Could you check a few things on this model? Use its own coordinates, in mm. Face numbers are marked on the shaded views. Round coordinates to 2 decimals unless told otherwise and drop trailing zeros. Write each loop counter-clockwise with the first axis right and the second up, starting at its lowest first coordinate (ties: lowest second). Pieces come first, ordered by that corner, then holes. Notation, with made-up numbers: (-2, 62.5) -> (32, 62.5) arc R15 cw to (32, 79.5) -> close; hole circle Ø4 at (61.25, 55). An arc over 180 degrees is marked (long way). Answer as CSV lines item,"result". Start each with the question number.
Q1. If I drill on line 1 (Y direction, x = -15.5, z = -14.5); line 2 (X direction, y = 8.75, z = -8); line 3 (Z direction, x = -18, y = 11.75), over which ranges is the centre line in solid material (lowest first)? Write a range as [from, to].
Q2. Will these pins go through, and if not, where does the flat tip stop? pin 1 Ø2 at (x, y) = (-8, 8.5) entering from -Z; pin 2 Ø1.9 at (y, z) = (-0.5, -1.5) entering from +X; pin 3 Ø18 at (x, z) = (0, 0) entering from +Y; pin 4 Ø2.5 at (x, z) = (8.84, 8.84) entering from -Y.
Q3. Imagine slicing it at A-A on z = 0. Please give me the cut outline in (x, y), and give its area (3 significant figures).
Q4. Imagine slicing it at C-C on y = 14.75. Please give me the cut outline in (x, z).
Q5. Imagine slicing it at B-B on x = 0. Please give me the cut outline in (y, z).
Q6. If we mould it in two halves opening along X, with no side actions, what happens to the marked faces 1, 2 and 3? For each: pulls with the +X half, pulls with the -X half, needs draft (parallel to the pull), parting line crosses it, or undercut.
from build123d import *
from build123d.topology import SkipClean

# Parameters (mm, degrees)
SKETCH_1_R          = 26
SKETCH_1_R_2        = 24
EXTRUDE_1_DEPTH     = 26
EXTRUDE_START       = 1
SKETCH_2_R          = 26
EXTRUDE_2_DEPTH     = 1
CUT_EXTRUDE_4_REACH = 47.033
FILLET_2_R          = 4
EXTRUDE_START_2     = 0.7
EXTRUDE_3_DEPTH     = 0.7
CUT_EXTRUDE_1_REACH = 48.036
SKETCH_4_R          = 7
HOLE_WIZARD_M31_D   = 3.4
CHAMFER_1_SIZE      = 0.5


with BuildPart() as part:
    # Эскиз1 → Бобышка-Вытянуть1 (new body)
    with BuildSketch(Plane(origin=(0, 0, 0), x_dir=(1, 0, 0), z_dir=(0, 1, 0))):
        with Locations(Location((0, 0, 0), (0, 0, 90))):
            Circle(SKETCH_1_R)
        with Locations(Location((0, 0, 0), (0, 0, 90))):
            Circle(SKETCH_1_R_2, mode=Mode.SUBTRACT)
    extrude(amount=EXTRUDE_1_DEPTH)

    # Эскиз2 → Бобышка-Вытянуть2 (add)
    with BuildSketch(Plane.XZ.offset(EXTRUDE_START)):
        with Locations(Location((0, 0, 0), (0, 0, 270))):
            Circle(SKETCH_2_R)
    extrude(amount=-EXTRUDE_2_DEPTH)

    # Эскиз9 → Вырез-Вытянуть4 (cut, up to next)
    with BuildSketch(Plane(origin=(0, 0, 0), x_dir=(1, 0, 0), z_dir=(0, 1, 0)), mode=Mode.PRIVATE) as cut_extrude_4_sk1:
        with BuildLine():
            Line((15, 18.734993995), (15, -18.734993995))
            ThreePointArc((15, -18.734993995), (24, 0), (15, 18.734993995))
        make_face()
    cut_extrude_4_tool1 = extrude(cut_extrude_4_sk1.sketch, amount=-CUT_EXTRUDE_4_REACH, mode=Mode.PRIVATE) & part.part
    add(cut_extrude_4_tool1.solids().sort_by_distance((18.66496, 0, 0))[0], mode=Mode.SUBTRACT)

    # Скругление2
    fillet_2_edges = [part.edges().sort_by_distance(p)[0] for p in [
        (15, -0.5, -18.734993995),
        (15, -0.5, 18.734993995),
    ]]
    fillet(fillet_2_edges, radius=FILLET_2_R)

    # Эскиз3 → Бобышка-Вытянуть3 (add)
    with SkipClean():  # the faces are left unmerged after this step: merging them gives an invalid solid
        with BuildSketch(Plane.XZ.offset(1).offset(EXTRUDE_START_2)):
            with BuildLine():
                Line((15, -6.244997998), (15, 6.244997998))
                ThreePointArc((15, 6.244997998), (16.303590006, 9.199549257), (19.364686571, 10.22833877))
                ThreePointArc((19.364686571, 10.22833877), (-21.9, 0), (19.364686571, -10.22833877))
                ThreePointArc((19.364686571, -10.22833877), (16.303590006, -9.199549257), (15, -6.244997998))
            make_face()
        extrude(amount=-EXTRUDE_3_DEPTH)

    # Эскиз4 → Вырез-Вытянуть1 (cut, up to next)
    with BuildSketch(Plane.XZ.offset(1.7), mode=Mode.PRIVATE) as cut_extrude_1_sk1:
        with Locations(Location((0, 0, 0), (0, 0, 270))):
            Circle(SKETCH_4_R)
    cut_extrude_1_tool1 = extrude(cut_extrude_1_sk1.sketch, amount=-CUT_EXTRUDE_1_REACH, mode=Mode.PRIVATE) & part.part
    add(cut_extrude_1_tool1.solids().sort_by_distance((0, -1.7, 0))[0], mode=Mode.SUBTRACT)

    # Отверстие с зазором M31 (through all)
    with Locations(Plane(origin=(0, -1.7, 0), x_dir=(-1, 0, 0), z_dir=(0, -1, 0))):
        with Locations((8.838834765, -8.838834765), (-8.838834765, -8.838834765), (-8.838834765, 8.838834765), (8.838834765, 8.838834765)):
            Hole(HOLE_WIZARD_M31_D / 2)

    # Фаска1
    chamfer_1_edges = [part.edges().sort_by_distance(p)[0] for p in [
        (0, -1, 26),
    ]]
    chamfer(chamfer_1_edges, length=CHAMFER_1_SIZE)


solid = part.part
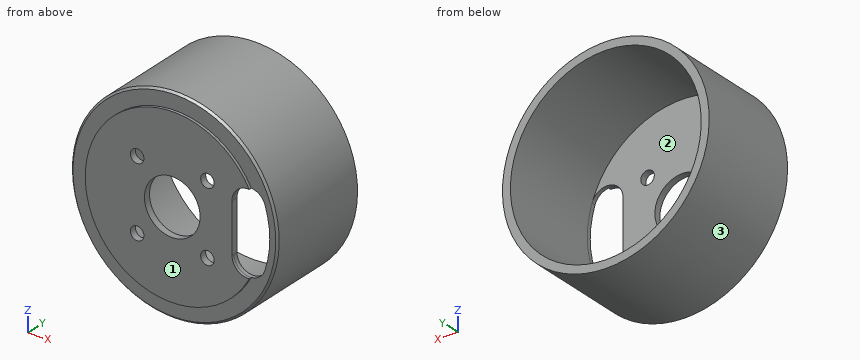
Checks:
1,line 1,"[-1.7, 0]"
1,line 2,"[-24.74, -22.63], [22.63, 24.74]"
1,line 3,"[-18.76, -15.87], [15.87, 18.76]"
2,pin 1,"z = -25.04"
2,pin 2,"x = 25.99"
2,pin 3,"y = 0"
2,pin 4,"through"
3,outline,"(-26, -0.5) -> (-25.5, -1) -> (-21.9, -1) -> (-21.9, -1.7) -> (-7, -1.7) -> (-7, 0) -> (-24, 0) -> (-24, 26) -> (-26, 26) -> close; (7, -1.7) -> (15, -1.7) -> (15, 0) -> (7, 0) -> close; (24, -1) -> (25.5, -1) -> (26, -0.5) -> (26, 26) -> (24, 26) -> close"
3,area,"149 mm^2"
4,outline,"circle Ø52 at (0, 0); hole circle Ø48 at (0, 0)"
5,outline,"(-1.7, -21.9) -> (-1, -21.9) -> (-1, -25.5) -> (-0.5, -26) -> (26, -26) -> (26, -24) -> (0, -24) -> (0, -7) -> (-1.7, -7) -> close; (-1.7, 7) -> (0, 7) -> (0, 24) -> (26, 24) -> (26, 26) -> (-0.5, 26) -> (-1, 25.5) -> (-1, 21.9) -> (-1.7, 21.9) -> close"
6,face 1,"needs draft"
6,face 2,"undercut"
6,face 3,"parting line crosses it"
